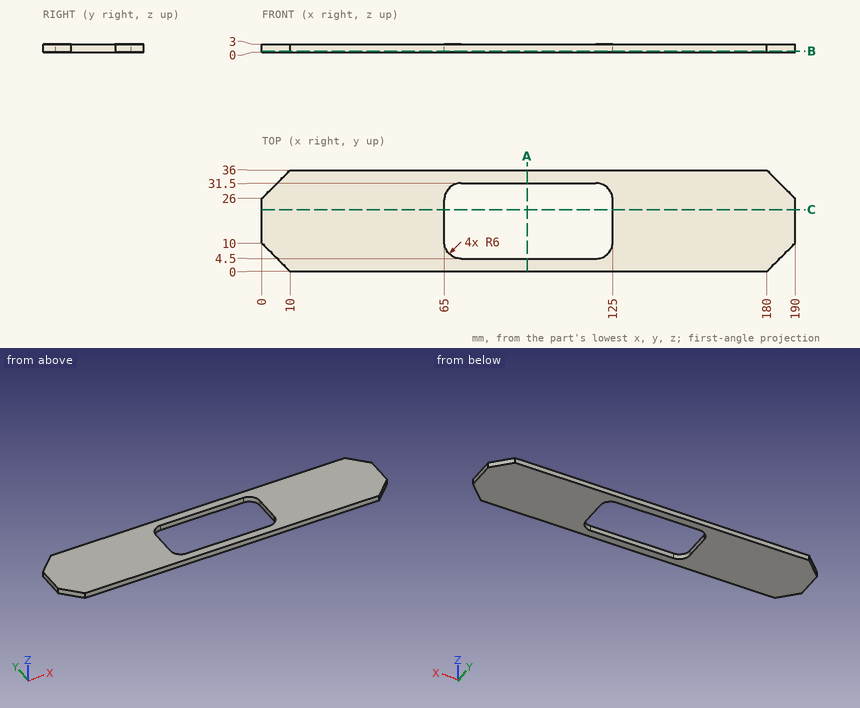
Can you work these out from the drawing? Everything is in mm from the part's minimum corner. Give positions to 0.01 mm unless a question says otherwise; leave off trailing zeros. Order: outer loops, then holes, each group sorted by start corner. A loop starts at its lowest first (then second) coordinate and runs counter-clockwise, first axis right, second up.
1. Suppose I cut it at C-C (y = 22). List the corners of the cut face in (x, z) for me, plus the area to 3 significant figures.
2. Suppose I cut it at A-A (x = 94.5). List the corners of the cut face in (y, z) for me.
3. Suppose I cut it at B-B (z = 0.5). List the corners of the cut face in (x, y) for me, plus the area to 3 significant figures.
4. I need wall thicknesses on L1, parallel to X at y = 17, z = 0.6; L2, parallel to Y at x = 102, z = 1.15; L3, parallel to Y at x = 70, z = 0.3. Which ranges of each line are inside material? Lowest first, please.
Solved:
1. outline: (0, 0) - (65, 0) - (65, 3) - (0, 3) - close; (125, 0) - (190, 0) - (190, 3) - (125, 3) - close
1. area: 390 mm2
2. outline: (0, 0) - (4.5, 0) - (4.5, 3) - (0, 3) - close; (31.5, 0) - (36, 0) - (36, 3) - (31.5, 3) - close
3. outline: (0, 10) - (10, 0) - (180, 0) - (190, 10) - (190, 26) - (180, 36) - (10, 36) - (0, 26) - close; hole (65, 10.5) arc R6 ccw to (71, 4.5) - (119, 4.5) arc R6 ccw to (125, 10.5) - (125, 25.5) arc R6 ccw to (119, 31.5) - (71, 31.5) arc R6 ccw to (65, 25.5) - close
3. area: 5,050 mm2
4. L1: x = 0 to 65, 125 to 190
4. L2: y = 0 to 4.5, 31.5 to 36
4. L3: y = 0 to 4.58, 31.42 to 36
